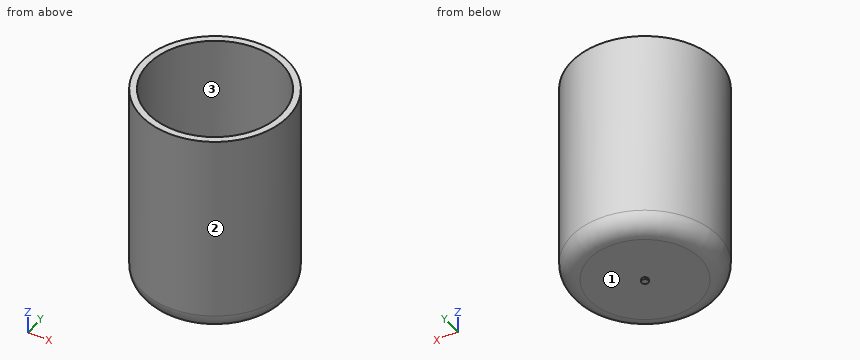
```python
from build123d import *

# Parameters (mm, degrees)
F2_R     = 1.5
F3_DEPTH = 1


with BuildPart() as f1:
    # F0 (on Front) → F1 (revolve)
    with BuildSketch(Plane.XZ):
        with BuildLine():
            Line((0, 3), (0, 0))
            Line((0, 0), (25, 0))
            ThreePointArc((25, 0), (30.656854, 2.343146), (33, 8))
            Line((33, 8), (33, 93))
            Line((33, 93), (30, 93))
            Line((30, 93), (30, 8))
            ThreePointArc((30, 8), (28.535534, 4.464466), (25, 3))
            Line((25, 3), (0, 3))
        make_face()
    revolve(axis=Axis((0, 0, 7.581016), (0, 0, 1)))

    # F2 (on face) → F3 (join)
    with BuildSketch(Plane(origin=(0, 0, 0), x_dir=(1, 0, 0), z_dir=(0, 0, -1))):
        Circle(F2_R)
    extrude(amount=F3_DEPTH)


solid = f1.part
```
Design review of the part built by this model. Coordinates are the model's own, in mm. Face numbers are marked on the shaded views. Round coordinates to 2 decimals unless told otherwise and drop trailing zeros. Order: outer loops, then holes, each group sorted by start corner. A loop starts at its lowest first (then second) coordinate and runs counter-clockwise, first axis right, second up. Notation, with made-up numbers: (29, -13) - (67, -13) arc R27 cw to (67, 5) - close; hole circle Ø11 at (33.5, 69.5). An arc over 180 degrees is marked (long way). Return JSON: item names as keys, results as strings.
Q1. Consider section C-C on z = 60. Write out the cut boundary in (x, y), plus the area to 3 significant figures.
Computed values:
{"outline": "circle Ø66 at (0, 0); hole circle Ø60 at (0, 0)", "area": "594 mm2"}
Q2. The part is to be moulded in two halves that separate along Y. For the marked faces 1, 2 and 3, say which applies: pulls with the +Y half, pulls with the -Y half, needs draft (parallel to the pull), parting line crosses it, or undercut.
Computed values:
{"face 1": "needs draft", "face 2": "parting line crosses it", "face 3": "undercut"}
Q3. For pin 1 Ø6 at (x, z) = (-17.5, 60.5) entering from +Y; pin 2 Ø15 at (x, y) = (-9, -12.5) entering from -Z; pin 3 Ø4 at (x, z) = (-7.5, 55) entering from -Y; pin 4 Ø12 at (y, z) = (-1, 60.5) entering from +X, all flat-tipped, find the tip position at first contact; note any pin that passes through.
Computed values:
{"pin 1": "stops at y = 29.64", "pin 2": "stops at z = 0", "pin 3": "stops at y = -32.54", "pin 4": "stops at x = 33"}
Q4. Wall thickness on L1, parallel to Y at x = 0, z = 32; L2, parallel to Z at x = -11, y = -4; L3, parallel to Y at x = 2, z = 12: over which ranges is each line inside the solid? List them lowest first. Write a range as [from, to].
Computed values:
{"L1": "y = [-33, -30], [30, 33]", "L2": "z = [0, 3]", "L3": "y = [-32.94, -29.93], [29.93, 32.94]"}
Q5. Consider section A-A on y = 0. Write out the cut boundary in (x, z), plus the area to 3 significant figures.
Computed values:
{"outline": "(-33, 8) arc R8 ccw to (-25, 0) - (-1.5, 0) - (-1.5, -1) - (1.5, -1) - (1.5, 0) - (25, 0) arc R8 ccw to (33, 8) - (33, 93) - (30, 93) - (30, 8) arc R5 cw to (25, 3) - (-25, 3) arc R5 cw to (-30, 8) - (-30, 93) - (-33, 93) - close", "area": "724 mm2"}
